```python
from build123d import *

# Parameters (mm, degrees)
F0_R     = 88.9
F0_R_2   = 6.35
F0_R_3   = 3.175
F1_DEPTH = 25.4


with BuildPart() as f1:
    # F0 (on Front) → F1 (new body)
    with BuildSketch(Plane.XZ):
        Circle(F0_R)
        with Locations((0, -76.2)):
            Circle(F0_R_2, mode=Mode.SUBTRACT)
        with Locations((38.1, -38.1)):
            Circle(F0_R_3, mode=Mode.SUBTRACT)
        with Locations((-76.2, 0)):
            Circle(F0_R_2, mode=Mode.SUBTRACT)
        with Locations((-38.1, 38.1)):
            Circle(F0_R_3, mode=Mode.SUBTRACT)
        with Locations((38.1, 38.1)):
            Circle(F0_R_3, mode=Mode.SUBTRACT)
        with Locations((76.2, 0)):
            Circle(F0_R_2, mode=Mode.SUBTRACT)
        with Locations((0, 76.2)):
            Circle(F0_R_2, mode=Mode.SUBTRACT)
    extrude(amount=F1_DEPTH)


solid = f1.part
```
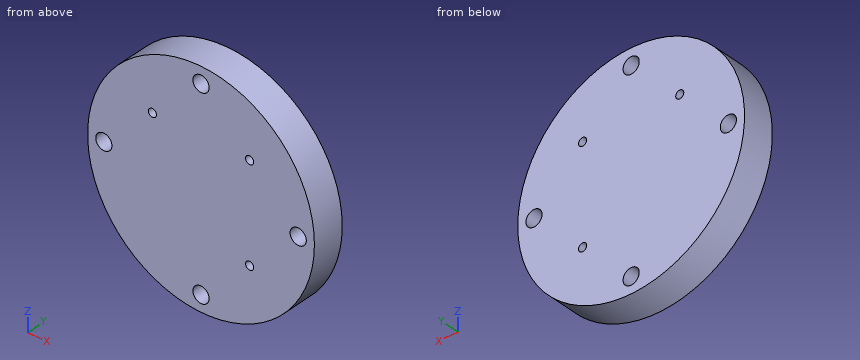
Input: part model. Units: mm. Frame: model coordinates. Coordinates: 2 decimals unless noted, no trailing zeros. Loops run counter-clockwise (first coordinate to the right, second up) from the corner with the lowest first, then second, coordinate; pieces in that order, holes last. Notation, with made-up numbers: (7.5, 60.25) - (22.5, 60.25) arc R16 ccw to (22.5, 86.25) - close; hole circle Ø9 at (-10.5, 10.25). An arc over 180 degrees is marked (long way). Answer in a Markdown table with one row per item.
(1) Cut plane D-D on x = 76.2. Output: boundary loops of the cut face in (y, z), plus the area to 3 significant figures.
Model answer:
| item | result |
|---|---|
| outline | (-25.4, -45.79) - (0, -45.79) - (0, -6.35) - (-25.4, -6.35) - close; (-25.4, 6.35) - (0, 6.35) - (0, 45.79) - (-25.4, 45.79) - close |
| area | 2,000 mm² |
(2) Cut plane C-C on z = -76.2. Output: boundary loops of the cut face in (x, y), plus the area to 3 significant figures.
Model answer:
| item | result |
|---|---|
| outline | (-45.79, -25.4) - (-6.35, -25.4) - (-6.35, 0) - (-45.79, 0) - close; (6.35, -25.4) - (45.79, -25.4) - (45.79, 0) - (6.35, 0) - close |
| area | 2,000 mm² |
(3) Material intervals for L1, parallel to Z at x = 3, y = -4.25; L2, parallel to Z at x = 38.1, y = -9.75 (3 decimals); L3, parallel to X at y = -7, z = 38, sorted ascending. Write a range as from..to.
Model answer:
| item | result |
|---|---|
| L1 | z = -88.85..-81.8, -70.6..70.6, 81.8..88.85 |
| L2 | z = -80.322..-41.275, -34.925..34.925, 41.275..80.322 |
| L3 | x = -80.37..-41.27, -34.93..34.93, 41.27..80.37 |
(4) Pin query (flat end, axial travel): P1, Ø3, axis at y = -20.5, z = -41, coming from the -X side; P2, Ø1.5, axis at x = 45, y = -8, coming from the +Z side; P3, Ø1, axis at x = 66.5, y = -6, coming from the -Z side. Return the tip coordinate at first contact, or that it passes through.
Model answer:
| item | result |
|---|---|
| P1 | stops at x = -79.64 |
| P2 | stops at z = 77.1 |
| P3 | stops at z = -59.56 |
(5) Cut plane B-B on x = 0. Output: boundary loops of the cut face in (y, z).
Model answer:
| item | result |
|---|---|
| outline | (-25.4, -88.9) - (0, -88.9) - (0, -82.55) - (-25.4, -82.55) - close; (-25.4, -69.85) - (0, -69.85) - (0, 69.85) - (-25.4, 69.85) - close; (-25.4, 82.55) - (0, 82.55) - (0, 88.9) - (-25.4, 88.9) - close |
(6) Cut plane A-A on y = -22.5. Output: boundary loops of the cut face in (x, z) (3 decimals), plus the area to 3 significant figures.
Model answer:
| item | result |
|---|---|
| outline | circle Ø177.8 at (0, 0); hole circle Ø12.7 at (-76.2, 0); hole circle Ø6.35 at (-38.1, 38.1); hole circle Ø12.7 at (0, -76.2); hole circle Ø12.7 at (0, 76.2); hole circle Ø6.35 at (38.1, -38.1); hole circle Ø6.35 at (38.1, 38.1); hole circle Ø12.7 at (76.2, 0) |
| area | 24,200 mm² |
